Can you work these out from the model? Positions are in its coordinate system, mm. A direction names the side the tool comes from. Give positions to 0.01 mm unless a question says otherwise; leave off trailing zeros. Loops run counter-clockwise (first coordinate to the right, second up) from the corner with the lowest first, then second, coordinate; pieces in that order, holes last. Notation, with made-up numbers: M 18,26.25 L 23,26.25 A14 cw 23,30.25 Z; hole C 81.25,53 d2. An arc over 180 degrees is marked long. Use CSV: the item, a comma, the result in double quotes.
from build123d import *

# Parameters (mm, degrees)
SKETCH_R        = 9.5
PAD_DEPTH       = 6
SKETCH001_R     = 9.5
PAD001_DEPTH    = 5
SKETCH002_R     = 4
POCKET_DEPTH    = 5
SKETCH003_R     = 2.5
SKETCH003_R_2   = 4
PAD002_DEPTH    = 4
SKETCH004_R     = 8.5
POCKET001_DEPTH = 4
PAD003_DEPTH    = 4


with BuildPart() as part:
    # Sketch → Pad (new body)
    with BuildSketch(Plane.XY):
        Circle(SKETCH_R)
        Polygon((3.752777, 6.5), (-3.752777, 6.5), (-7.505553, 0), (-3.752777, -6.5), (3.752777, -6.5), (7.505553, 0), align=None, mode=Mode.SUBTRACT)
    extrude(amount=PAD_DEPTH)

    # Sketch001 (on Face9 of Pad) → Pad001 (join)
    with BuildSketch(Plane.XY.offset(6)):
        Circle(SKETCH001_R)
    extrude(amount=PAD001_DEPTH)

    # Sketch002 (on Face10 of Pad001) → Pocket (cut)
    with BuildSketch(Plane.XY.offset(11)):
        Circle(SKETCH002_R)
    extrude(amount=-POCKET_DEPTH, mode=Mode.SUBTRACT)

    # Sketch003 (on Face10 of Pocket) → Pad002 (join)
    with BuildSketch(Plane.XY.offset(11)):
        with BuildLine():
            ThreePointArc((0, 9.5), (-9.5, 0), (0, -9.5))
            Line((0, -9.5), (80, -9.5))
            ThreePointArc((80, -9.5), (89.5, 0), (80, 9.5))
            Line((0, 9.5), (80, 9.5))
        make_face()
        with Locations((80, 0)):
            Circle(SKETCH003_R, mode=Mode.SUBTRACT)
        Circle(SKETCH003_R_2, mode=Mode.SUBTRACT)
    extrude(amount=PAD002_DEPTH)

    # Sketch004 (on Face17 of Pad002) → Pocket001 (cut)
    with BuildSketch(Plane.XY.offset(15)):
        Circle(SKETCH004_R)
    extrude(amount=-POCKET001_DEPTH, mode=Mode.SUBTRACT)

    # Sketch005 (on Face10 of Pocket001) → Pad003 (join)
    with BuildSketch(Plane(origin=(0, 0, 11), x_dir=(1, 0, 0), z_dir=(0, 0, -1))):
        with BuildLine():
            ThreePointArc((8.87412, -9.5), (13, 0), (8.87412, 9.5))
            Line((0, 9.5), (8.87412, 9.5))
            ThreePointArc((0, -9.5), (9.5, 0), (0, 9.5))
            Line((0, -9.5), (8.87412, -9.5))
        make_face()
    extrude(amount=PAD003_DEPTH)


solid = part.part
Q1. I want a section at D-D, the plane z = 10. Please give me the cut outline in (x, y).
Model answer:
outline,"M 0,-9.5 L 8.87,-9.5 A13 ccw 8.87,9.5 L 0,9.5 A9.5 ccw Z; hole C 0,0 d8"
Q2. If we mould it in two halves opening along Y, with no side actions, what happens to faces 4 (the cylindrical face through (89.498, -0.209, 12.972)), 5 (the flat face through (50, 0, 15)), 6 (the flat face through (3, -3, 6)), 7 (the flat face through (0, -6.5, 3))? For each: released by +Y, released by -Y, zero draft, split by the parting line, or undercut.
Model answer:
face 4,"split by the parting line"
face 5,"zero draft"
face 6,"undercut"
face 7,"undercut"
Q3. I'm going to push flat-ended pins straight in: P1, Ø9.5, axis at x = 53, y = -1, coming from the -Z side; P2, Ø10.5, axis at x = 0, y = 0, coming from the -Z side; P3, Ø1, axis at y = 2.5, z = 6, coming from the +X side; P4, Ø4, axis at x = 12.5, z = 2.5, coming from the -Y side. Where does each tip first touch, or does it pass through?
Model answer:
P1,"z = 11"
P2,"z = 6"
P3,"x = 9.29"
P4,"through"
Q4. I want a section at B-B, the plane y = 1.5. Please give me the cut outline in (x, z), then the cut area to 3 significant figures.
Model answer:
outline,"M -9.38,0 L -6.64,0 L -6.64,6 L -3.71,6 L -3.71,11 L -8.37,11 L -8.37,15 L -9.38,15 Z; M 3.71,6 L 6.64,6 L 6.64,0 L 9.38,0 L 9.38,7 L 12.91,7 L 12.91,11 L 78,11 L 78,15 L 8.37,15 L 8.37,11 L 3.71,11 Z; M 82,11 L 89.38,11 L 89.38,15 L 82,15 Z"
area,"416 mm2"
Q5. I want a section at A-A, the plane z = 2.5. Please give me the cut outline in (x, y).
Model answer:
outline,"C 0,0 d19; hole M -7.51,0 L -3.75,-6.5 L 3.75,-6.5 L 7.51,0 L 3.75,6.5 L -3.75,6.5 Z"
Q6. For faces 1 (the flat face through (-5.66, -3.2, 2.96)), 2 (the cylindrical face through (4.57, 7.167, 13.028)), 3 (the cylindrical face through (13, 0, 9)), which set-ups out of +Z, -Z, +X, -X, +Y, -Y let a thin tool reach every point of the face, with its end or its side?
Model answer:
face 1,"-Z"
face 2,"+Z"
face 3,"-Z, +X"
Q7. Please list where these lines run through material, in increasing order: L1, parallel to Y at x = 0, z = 9.2; L2, parallel to X at y = 0.75, z = 12; L3, parallel to Y at x = 0, z = 12.5. Write a range as from..to.
Model answer:
L1,"-9.5..-4, 4..9.5"
L2,"-9.47..-8.47, 8.47..77.62, 82.38..89.47"
L3,"-9.5..-8.5, 8.5..9.5"
Q8. I want a section at C-C, the plane x = 6.5. Please give me the cut outline in (y, z).
Model answer:
outline,"M -9.5,7 L -6.93,7 L -6.93,0 L -1.74,0 L -1.74,6 L 1.74,6 L 1.74,0 L 6.93,0 L 6.93,7 L 9.5,7 L 9.5,15 L 5.48,15 L 5.48,11 L -5.48,11 L -5.48,15 L -9.5,15 Z"
